CAD build for the part. Positions are in the model's coordinates, mm. Face numbers are marked on the shaded views. A direction names the side the tool comes from. Give positions to 0.01 mm unless a question says otherwise; leave off trailing zeros. Order: outer loops, then holes, each group sorted by start corner. A loop starts at its lowest first (then second) coordinate and runs counter-clockwise, first axis right, second up.
Item 1: Band-saw the part on A-A on z = 0. Give the cut face in (x, y).
Item 2: Band-saw the part on D-D on y = 71.5. Give the cut face in (x, z).
Item 3: Flat gauge pins, fed straight in: P1, Ø12, axis at x = 40.5, y = 27.5, coming from the +Z side; P2, Ø8, axis at y = 75.5, z = 20, coming from the +X side; P3, Ø1, axis at x = 38.5, y = 53.5, coming from the +Z side. Where does each tip first touch, or does it go through?
Item 4: Band-saw the part on B-B on x = 0. Give the cut face in (y, z).
Item 5: Wall check: L1, parallel to Y at x = -16, z = -49.5; L2, parallel to Z at x = 12.5, y = 17; L3, parallel to Z at x = 33, y = 97. Give the ranges that are in metal, low to high.
Item 6: Band-saw the part on C-C on y = 105. Give the cut face in (x, z).
Item 7: Two-plate mould, pull along Z, no slides. Class the marked faces 4, 5 and 6: released by +Z, released by -Z, zero draft, split by the parting line, or undercut.
Item 8: Which spindle directions (+Z, -Z, +X, -X, +Y, -Y) get a long thin tool onto all of the face, cutting with end or side? Do the marked faces 1, 2 and 3. Say none if no direction does.
```python
from build123d import *

# Parameters (mm, degrees)
BOSS_EXTRUDE1_START = 6.35
SKETCH2_R           = 70
SKETCH2_R_2         = 55
BOSS_EXTRUDE1_DEPTH = 6.35
SKETCH5_W           = 76.2
SKETCH5_H           = 76.2
BOSS_EXTRUDE3_DEPTH = 76.2


with BuildPart() as part:
    # Sketch1 → Revolve1 (revolve)
    with BuildSketch(Plane.XY, mode=Mode.PRIVATE) as revolve1_sk:
        with BuildLine():
            Line((55, 0), (55, 76.2))
            Line((55, 76.2), (70, 76.2))
            ThreePointArc((70, 76.2), (60.645745066, 38.609228172), (57.5, 0))
            Line((57.5, 0), (55, 0))
        make_face()
    revolve(revolve1_sk.sketch.rotate(Axis((0, 0, 0), (0, 1, 0)), 90), axis=Axis((0, 0, 0), (0, 1, 0)))

    # Sketch2 → Boss-Extrude1 (add)
    # profile 1 of 2: a face of its own
    with BuildSketch(Plane(origin=(0, 76.2, 0), x_dir=(1, 0, 0), z_dir=(0, 1, 0)).offset(BOSS_EXTRUDE1_START)):
        with Locations(Location((0, 0, 0), (0, 0, 270))):
            Circle(SKETCH2_R)
        with Locations(Location((0, 0, 0), (0, 0, 90))):
            Circle(SKETCH2_R_2, mode=Mode.SUBTRACT)
    # profile 2 of 2: a face of its own
    with BuildSketch(Plane(origin=(0, 76.2, 0), x_dir=(1, 0, 0), z_dir=(0, 1, 0)).offset(BOSS_EXTRUDE1_START)):
        with Locations(Location((0, 0, 0), (0, 0, 90))):
            Circle(SKETCH2_R_2)
    extrude(amount=-BOSS_EXTRUDE1_DEPTH)

    # Sketch5 → Boss-Extrude3 (add)
    with BuildSketch(Plane(origin=(0, 82.55, 0), x_dir=(1, 0, 0), z_dir=(0, 1, 0))):
        Rectangle(SKETCH5_W, SKETCH5_H)
    extrude(amount=BOSS_EXTRUDE3_DEPTH)


solid = part.part
```
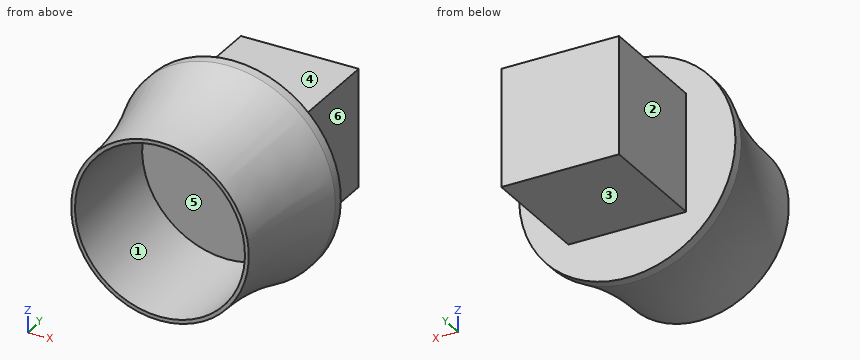
The answers:
1. outline: (-70, 76.2) arc R238.51 cw to (-57.5, 0) - (-55, 0) - (-55, 76.2) - (55, 76.2) - (55, 0) - (57.5, 0) arc R238.51 cw to (70, 76.2) - (70, 82.55) - (38.1, 82.55) - (38.1, 158.75) - (-38.1, 158.75) - (-38.1, 82.55) - (-70, 82.55) - close
2. outline: circle Ø136.94 at (0, 0); hole circle Ø110 at (0, 0)
3. P1: stops at z = 48.06
3. P2: stops at x = 68.13
3. P3: stops at z = 51
4. outline: (0, -57.5) arc R238.51 cw to (76.2, -70) - (82.55, -70) - (82.55, -38.1) - (158.75, -38.1) - (158.75, 38.1) - (82.55, 38.1) - (82.55, 70) - (76.2, 70) arc R238.51 cw to (0, 57.5) - (0, 55) - (76.2, 55) - (76.2, -55) - (0, -55) - close
5. L1: y = 76.2 to 82.55
5. L2: z = -56.75 to -53.56, 53.56 to 56.75
5. L3: z = -38.1 to 38.1
6. outline: (-38.1, -38.1) - (38.1, -38.1) - (38.1, 38.1) - (-38.1, 38.1) - close
7. face 4: released by +Z
7. face 5: undercut
7. face 6: zero draft
8. face 1: -Y
8. face 2: +Z, -Z, -X, +Y
8. face 3: -Z, +X, -X, +Y
